Source: CAD feature listing. Evaluate the final solid. Frame: model axes, mm. A direction names the side the tool comes from. Coordinates: 2 decimals unless noted, no trailing zeros. Write each loop counter-clockwise with the first axis right and the second up, starting at its lowest first coordinate (ties: lowest second). Pieces come first, ordered by that corner, then holes. Notation, with made-up numbers: (12.25, 80) -> (62.25, 80) arc R32 cw to (62.25, 106) -> close; hole circle Ø9 at (16, 4). An arc over 180 degrees is marked (long way). Write item = value, one per line.
from build123d import *

# Parameters (mm, degrees)
SKETCH1_W               = 38.7
SKETCH1_H               = 51.5
BOSS_EXTRUDE1_DEPTH     = 8
SKETCH2_R               = 1.5
CUT_EXTRUDE1_DEPTH      = 9
SKETCH6_W               = 25
SKETCH6_H               = 13
BOSS_EXTRUDE3_DEPTH     = 2
CUT_EXTRUDE2_START      = -9
SKETCH3_R               = 2.75
CUT_EXTRUDE2_DEPTH      = 12
MIRROR3_START           = -9
MIRROR3_COPY_1_SKETCH_R = 2.75
MIRROR3_COPY_1_DEPTH    = 12
SKETCH4_R               = 2.75
CUT_EXTRUDE3_DEPTH      = 3
CUT_EXTRUDE3_DEPTH_BACK = 9
FILLET1_R               = 2
FILLET2_R               = 2


with BuildPart() as part:
    # Sketch1 → Boss-Extrude1 (new body)
    with BuildSketch(Plane(origin=(0, 0, 0), x_dir=(1, 0, 0), z_dir=(0, 1, 0))):
        Rectangle(SKETCH1_W, SKETCH1_H)
    extrude(amount=BOSS_EXTRUDE1_DEPTH)

    # Sketch2 → Cut-Extrude1 (cut, through all)
    with BuildSketch(Plane(origin=(0, 8, 0), x_dir=(1, 0, 0), z_dir=(0, 1, 0))):
        with Locations((11.65, 10.75)):
            Circle(SKETCH2_R)
        with Locations((-13.35, 10.75)):
            Circle(SKETCH2_R)
    cut_extrude1 = extrude(amount=-CUT_EXTRUDE1_DEPTH, mode=Mode.SUBTRACT)

    # Mirror1: Cut-Extrude1 across plane
    add(cut_extrude1.mirror(Plane.XY), mode=Mode.SUBTRACT)

    # Sketch6 → Boss-Extrude3 (add)
    with BuildSketch(Plane(origin=(0, 8, 0), x_dir=(1, 0, 0), z_dir=(0, 1, 0))):
        with Locations((-6.85, -19.25)):
            Rectangle(SKETCH6_W, SKETCH6_H)
    extrude(amount=BOSS_EXTRUDE3_DEPTH)

    # Sketch3 → Cut-Extrude2 (cut)
    with BuildSketch(Plane(origin=(0, 8, 0), x_dir=(1, 0, 0), z_dir=(0, 1, 0)).offset(CUT_EXTRUDE2_START)):
        with Locations((13.35, -19.25)):
            Circle(SKETCH3_R)
    cut_extrude2 = extrude(amount=CUT_EXTRUDE2_DEPTH, mode=Mode.SUBTRACT)

    # Mirror2: Cut-Extrude2 across plane
    add(cut_extrude2.mirror(Plane(origin=(0, 0, 0), x_dir=(0, 0, 1), z_dir=(1, 0, 0))), mode=Mode.SUBTRACT)

    # Mirror3: Cut-Extrude2 across plane
    add(cut_extrude2.mirror(Plane.XY), mode=Mode.SUBTRACT)

    # Mirror3 copy 1 sketch → Mirror3 copy 1 (cut)
    with BuildSketch(Plane(origin=(0, 8, 0), x_dir=(-1, 0, 0), z_dir=(0, 1, 0)).offset(MIRROR3_START)):
        with Locations((13.35, -19.25)):
            Circle(MIRROR3_COPY_1_SKETCH_R)
    extrude(amount=MIRROR3_COPY_1_DEPTH, mode=Mode.SUBTRACT)

    # Sketch4 → Cut-Extrude3 (cut, two sides)
    with BuildSketch(Plane(origin=(0, 8, 0), x_dir=(1, 0, 0), z_dir=(0, 1, 0))) as cut_extrude3_sk:
        with Locations((0, 19.25)):
            Circle(SKETCH4_R)
    extrude(amount=CUT_EXTRUDE3_DEPTH, mode=Mode.SUBTRACT)
    extrude(cut_extrude3_sk.sketch, amount=-CUT_EXTRUDE3_DEPTH_BACK, mode=Mode.SUBTRACT)

    # Fillet1
    fillet1_edges = [part.edges().sort_by_distance(p)[0] for p in [
        (5.65, 9, 25.75),
        (5.65, 9, 12.75),
        (-19.35, 9, 12.75),
    ]]
    fillet(fillet1_edges, radius=FILLET1_R)

    # Fillet2
    fillet2_edges = [part.edges().sort_by_distance(p)[0] for p in [
        (19.35, 4, 25.75),
        (-19.35, 5, 25.75),
        (-19.35, 4, -25.75),
        (19.35, 4, -25.75),
    ]]
    fillet(fillet2_edges, radius=FILLET2_R)


solid = part.part
1) Cut plane D-D, the plane z = -19.25. Output: boundary loops of the cut face in (x, y), and give its area (3 significant figures).
Answer block:
outline = (-19.35, 0) -> (-16.1, 0) -> (-16.1, 8) -> (-19.35, 8) -> close; (-10.6, 0) -> (-2.75, 0) -> (-2.75, 8) -> (-10.6, 8) -> close; (2.75, 0) -> (10.6, 0) -> (10.6, 8) -> (2.75, 8) -> close; (16.1, 0) -> (19.35, 0) -> (19.35, 8) -> (16.1, 8) -> close
area = 178 mm2
2) Cut plane A-A, the plane z = -10.75. Output: boundary loops of the cut face in (x, y), and give its area (3 significant figures).
Answer block:
outline = (-19.35, 0) -> (-14.85, 0) -> (-14.85, 8) -> (-19.35, 8) -> close; (-11.85, 0) -> (10.15, 0) -> (10.15, 8) -> (-11.85, 8) -> close; (13.15, 0) -> (19.35, 0) -> (19.35, 8) -> (13.15, 8) -> close
area = 262 mm2
3) Cut plane B-B, the plane x = 0. Output: boundary loops of the cut face in (y, z).
Answer block:
outline = (0, -25.75) -> (8, -25.75) -> (8, -22) -> (0, -22) -> close; (0, -16.5) -> (8, -16.5) -> (8, 12.75) -> (10, 12.75) -> (10, 25.75) -> (0, 25.75) -> close
4) Cut plane C-C, the plane y = 6.5. Give the number of separate pieces and of enclosed holes in the cut face, and give its area (3 significant figures).
Answer block:
separate_pieces = 1
enclosed_holes = 9
area = 1,840 mm2
5) Reachability of faces 1 (the cylindrical face through (-12.992, 3.944, -16.523)), 2 (the cylindrical face through (-18.78, 9.01, 13.35)) from +Z, -Z, +X, -X, +Y, -Y: full face, straight path, thin tool, end or side. Return the list, or none.
Answer block:
face_1 = +Y, -Y
face_2 = -Z, -X, +Y
6) Pull-direction query (X, two-part tool) for faces 3 (the cylindrical face through (10.15, 4.06, 10.82)), 4 (the cylindrical face through (-14.85, 4.06, 10.82)), 5 (the flat face through (-7, 9, 12.75)), 6 (the cylindrical face through (5.05, 9.01, 25.18)); classes: +X half, -X half, draft (parallel to the pull), parting line (faces both ways), or undercut.
Answer block:
face_3 = undercut
face_4 = undercut
face_5 = draft
face_6 = +X half
7) Material intervals for probe 1 along X at (y, z) = (3, 10.75); probe 2 along X at (y, z) = (2.5, -9.5); probe 3 along Y at (x, z) = (-12, -14), sorted ascending. Write a range as [from, to].
Answer block:
probe_1 = [-19.35, -14.85], [-11.85, 10.15], [13.15, 19.35]
probe_2 = [-19.35, -14.18], [-12.52, 10.82], [12.48, 19.35]
probe_3 = [0, 8]
8) First-contact query: pin 1 Ø10 at (x, z) = (9.5, 17) entering from -Y; pin 2 Ø2.5 at (x, z) = (11.65, 10.75) entering from -Y; pin 3 Ø9 at (x, z) = (-13.35, -19.25) entering from +Y; pin 4 Ø1.6 at (y, z) = (9, 19) entering from +X. Flat tips, straight axial feed; report the tip coordinate or a pass-through.
Answer block:
pin_1 = 0
pin_2 = through
pin_3 = 8
pin_4 = 5.65
